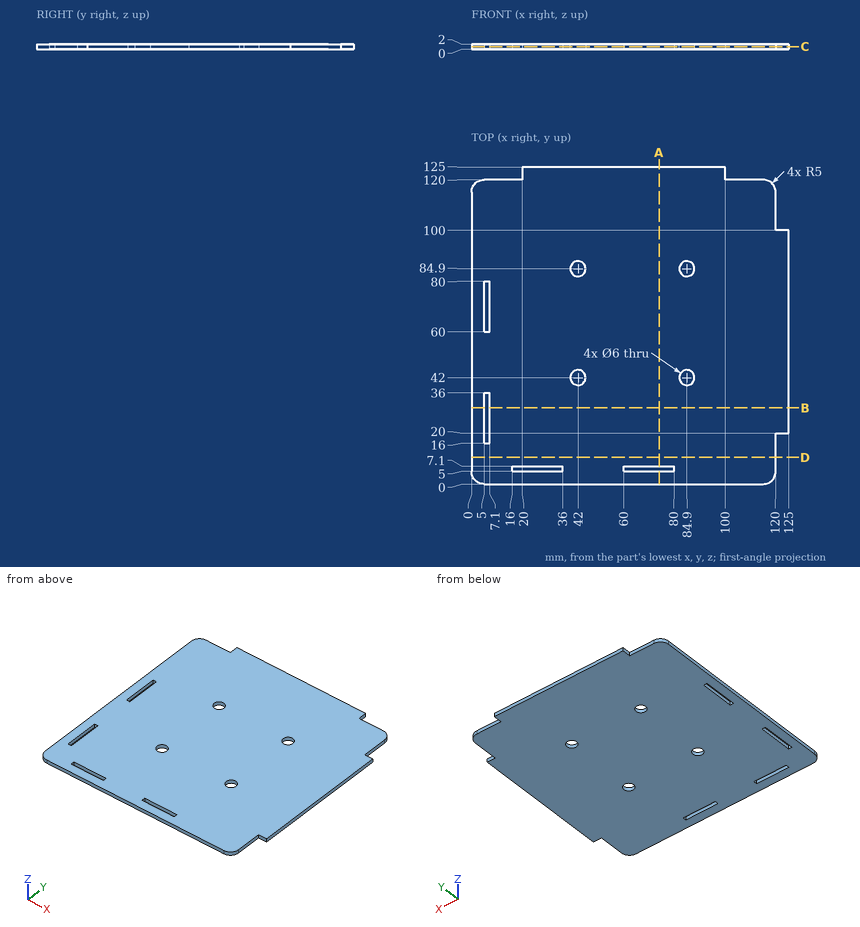
The drawing under review shows one solid part. Ordinate dimensions are in mm from its lowest x, y, z. Round coordinates to 2 decimals unless told otherwise and drop trailing zeros. Loops run counter-clockwise (first coordinate to the right, second up) from the corner with the lowest first, then second, coordinate; pieces in that order, holes last. Notation, with made-up numbers: (75.25, -24) - (92.25, -24) arc R22 ccw to (92.25, 3) - close; hole circle Ø4 at (56.25, -24). An arc over 180 degrees is marked (long way). One line per question, with ' | ' between items.
1. We need section C-C, the plane z = 0.95. State how many separate pieces and enclosed holes the cut face has, and give its area (3 significant figures).
Results are:
separate pieces: 1 | enclosed holes: 8 | area: 14,900 mm²
2. For L1, parallel to Y at x = 84.9, z = 1.25; L2, parallel to X at y = 44, z = 0.35; L3, parallel to Y at x = 17.5, z = 1.2, list the stretches that pass through material, from the lowest coordinate up. Write a range as [from, to].
Results are:
L1: y = [0, 39], [45, 81.9], [87.9, 125] | L2: x = [0, 39.76], [44.24, 82.66], [87.14, 125] | L3: y = [0, 5], [7.1, 120]
3. We need section D-D, the plane y = 10.5. State the section outline as (x, z) points, and give its area (3 significant figures).
Results are:
outline: (0, 0) - (120, 0) - (120, 2) - (0, 2) - close | area: 240 mm²
4. We need section A-A, the plane x = 74. State the section outline as (y, z) points.
Results are:
outline: (0, 0) - (5, 0) - (5, 2) - (0, 2) - close; (7.1, 0) - (125, 0) - (125, 2) - (7.1, 2) - close
5. Clearance check with flat-ended pins moving along their axes: P1, Ø3.5, axis at x = 84.9, y = 42, coming from the +Z side; P2, Ø0.6, axis at x = 123, z = 1.5, coming from the -Y side; P3, Ø1, axis at x = 6, z = 1, coming from the +Y side. State where each tip first meets the part, or that it passes through.
Results are:
P1: passes through | P2: stops at y = 20 | P3: stops at y = 120
